```python
from build123d import *

# Parameters (mm, degrees)
MODEL_R         = 1
MODEL_R_2       = 1.05
MODEL_W         = 13.99947
MODEL_H         = 13.99944
MODEL_W_2       = 2.54
MODEL_H_2       = 5.78308735
MODEL_W_3       = 13.9994
MODEL_W_4       = 13.9993
MODEL_H_3       = 13.9993
MODEL_R_3       = 2.032
MODEL_R_4       = 3.048
EXTRUDE_1_DEPTH = 1.5


with BuildPart() as part:
    # Model → 凸台-拉伸1 (new body)
    with BuildSketch(Plane.XY):
        with BuildLine():
            Line((57.046434605, 41.37894176), (0.354810268, 41.37894176))
            ThreePointArc((0.354810268, 41.37894176), (-0.846923686, 40.881370762), (-1.345189448, 39.679924707))
            Line((-1.345189448, 39.679924707), (-1.353515518, 25.280051374))
            Line((-1.353515518, 25.280051374), (-1.356811329, 19.579970423))
            Line((-1.356811329, 19.579970423), (-4.853485523, 18.100805857))
            Line((-4.853485523, 18.100805857), (-4.853710523, 15.920120221))
            Line((-4.853710523, 15.920120221), (-4.853736766, 15.66577888))
            Line((-4.853736766, 15.66577888), (-1.359820188, 14.394107598))
            Line((-1.359820188, 14.394107598), (-1.362991715, 8.917997305))
            Line((-1.362991715, 8.917997305), (-4.9049154, 4.538497879))
            Line((-4.9049154, 4.538497879), (-4.9049154, 3.15597541))
            Line((-4.9049154, 3.15597541), (-4.883883595, 2.639206616))
            Line((-4.883883595, 2.639206616), (-4.813264805, 2.011073476))
            Line((-4.813264805, 2.011073476), (-4.687062167, 1.387481119))
            Line((-4.687062167, 1.387481119), (-4.516803943, 0.776764684))
            Line((-4.516803943, 0.776764684), (-4.295659415, 0.187060206))
            Line((-4.295659415, 0.187060206), (-4.03681533, -0.378036856))
            Line((-4.03681533, -0.378036856), (-3.730362364, -0.921623746))
            Line((-3.730362364, -0.921623746), (-3.390574278, -1.434889052))
            Line((-3.390574278, -1.434889052), (-2.992281832, -1.942165148))
            Line((-2.992281832, -1.942165148), (-2.558331876, -2.409802006))
            Line((-2.558331876, -2.409802006), (-2.102251702, -2.829663369))
            Line((-2.102251702, -2.829663369), (-1.614610519, -3.215411153))
            Line((-1.614610519, -3.215411153), (-1.088890304, -3.567123565))
            Line((-1.088890304, -3.567123565), (-0.532800957, -3.878547051))
            Line((-0.532800957, -3.878547051), (0.038326794, -4.140153507))
            Line((0.038326794, -4.140153507), (0.615600502, -4.353028424))
            Line((0.615600502, -4.353028424), (1.223529929, -4.526191258))
            Line((1.223529929, -4.526191258), (1.847223482, -4.64943937))
            Line((1.847223482, -4.64943937), (2.464503115, -4.722060038))
            Line((2.464503115, -4.722060038), (2.992774524, -4.743685))
            Line((2.992774524, -4.743685), (54.34686609, -4.743685))
            Line((54.34686609, -4.743685), (54.87843401, -4.722059086))
            Line((54.87843401, -4.722059086), (55.492240411, -4.649391053))
            Line((55.492240411, -4.649391053), (56.11599848, -4.526806688))
            Line((56.11599848, -4.526806688), (56.726168878, -4.352867841))
            Line((56.726168878, -4.352867841), (57.302144081, -4.140491025))
            Line((57.302144081, -4.140491025), (57.880206411, -3.875955859))
            Line((57.880206411, -3.875955859), (58.434482529, -3.563431063))
            Line((58.434482529, -3.563431063), (58.947571314, -3.220379587))
            Line((58.947571314, -3.220379587), (59.445938304, -2.8287768))
            Line((59.445938304, -2.8287768), (59.905767444, -2.401934126))
            Line((59.905767444, -2.401934126), (60.332973054, -1.941418241))
            Line((60.332973054, -1.941418241), (60.721224007, -1.446690794))
            Line((60.721224007, -1.446690794), (61.064717919, -0.934798534))
            Line((61.064717919, -0.934798534), (61.379380282, -0.376374826))
            Line((61.379380282, -0.376374826), (61.644240363, 0.202684675))
            Line((61.644240363, 0.202684675), (61.855333273, 0.776565869))
            Line((61.855333273, 0.776565869), (62.029241049, 1.384922025))
            Line((62.029241049, 1.384922025), (62.152356641, 2.011350393))
            Line((62.152356641, 2.011350393), (62.226202972, 2.636734827))
            Line((62.226202972, 2.636734827), (62.245297192, 3.166071528))
            Line((62.245297192, 3.166071528), (58.745412398, 6.86443549))
            Line((58.745412398, 6.86443549), (58.74568075, 14.685402523))
            Line((58.74568075, 14.685402523), (62.245579127, 15.434705638))
            Line((62.245579127, 15.434705638), (62.245861062, 18.167199282))
            Line((62.245861062, 18.167199282), (58.745799684, 19.296928449))
            Line((58.745799684, 19.296928449), (58.745975132, 24.929084585))
            Line((58.745975132, 24.929084585), (58.746434604, 39.678888803))
            ThreePointArc((58.746434604, 39.678888803), (58.248534856, 40.881004565), (57.046434605, 41.37894176))
        make_face()
        with Locations((8.744501265, -2.189788582)):
            Circle(MODEL_R, mode=Mode.SUBTRACT)
        with Locations((19.14575, 5.311768186)):
            Circle(MODEL_R_2, mode=Mode.SUBTRACT)
        with Locations((9.620765, 9.78198)):
            Rectangle(MODEL_W, MODEL_H, mode=Mode.SUBTRACT)
        with Locations((-2.255498735, 16.910211418)):
            Circle(MODEL_R, mode=Mode.SUBTRACT)
        with Locations((19.167580955, 11.605191102)):
            Rectangle(MODEL_W_2, MODEL_H_2, mode=Mode.SUBTRACT)
        with Locations((38.19575, 5.272237591)):
            Circle(MODEL_R_2, mode=Mode.SUBTRACT)
        with Locations((48.744501265, -2.189788582)):
            Circle(MODEL_R, mode=Mode.SUBTRACT)
        with Locations((28.6707, 9.78198)):
            Rectangle(MODEL_W_3, MODEL_H, mode=Mode.SUBTRACT)
        with Locations((47.72075, 9.78198)):
            Rectangle(MODEL_W_4, MODEL_H, mode=Mode.SUBTRACT)
        with Locations((59.944501265, 16.910211418)):
            Circle(MODEL_R, mode=Mode.SUBTRACT)
        with Locations((9.620765, 28.83195)):
            Rectangle(MODEL_W, MODEL_H_3, mode=Mode.SUBTRACT)
        with Locations((19.1458, 28.832)):
            Circle(MODEL_R_3, mode=Mode.SUBTRACT)
        with Locations((0.354810268, 39.67894176)):
            Circle(MODEL_R, mode=Mode.SUBTRACT)
        with Locations((19.14575, 33.310608186)):
            Circle(MODEL_R_2, mode=Mode.SUBTRACT)
        with Locations((28.6708, 28.832)):
            Circle(MODEL_R_4, mode=Mode.SUBTRACT)
        with Locations((38.1958, 28.832)):
            Circle(MODEL_R_3, mode=Mode.SUBTRACT)
        with Locations((47.72075, 28.83195)):
            Rectangle(MODEL_W_4, MODEL_H_3, mode=Mode.SUBTRACT)
        with Locations((38.194579287, 33.311869349)):
            Circle(MODEL_R_2, mode=Mode.SUBTRACT)
        with Locations((57.046434605, 39.67894176)):
            Circle(MODEL_R, mode=Mode.SUBTRACT)
    extrude(amount=EXTRUDE_1_DEPTH)


solid = part.part
```
Read the model definition and answer for the solid it produces. Units are mm, in the model's axes. A direction names the side the tool comes from. Give positions to 0.01 mm unless a question says otherwise; leave off trailing zeros. Loops run counter-clockwise (first coordinate to the right, second up) from the corner with the lowest first, then second, coordinate; pieces in that order, holes last.
Item 1: For faces 5 (the cylindrical face through (58.26, 40.87, 0.74)), 6 (the flat face through (40.721, 29, 1)), 7 (the flat face through (-3.13, 15.04, 0.74)), determine the directions among +Z, -Z, +X, -X, +Y, -Y from which every point of the face is accessible in a straight line to the end or side of a thin tool.
Item 2: The part is cut by section C-C (y = 23.5). Write down the section's boundary in (x, z).
Item 3: The part is cut by section B-B (x = 13.5). Write down the section's boundary in (y, z).
Item 4: Find the intervals of material crossed by line 1 along Y through (x, z) = (41.5, 0.1); line 2 along X through (y, z) = (22.5, 0.6); line 3 along X through (y, z) = (11, 0.25), in increasing order.
Item 5: The part is cut by section D-D (y = 8). Write down the section's boundary in (x, z), and give its area (3 significant figures).
Item 6: The mould has two halves that part along X. Classify faces 1 (the flat face through (60.471, 15.055, 0.74)), 2 (the cylindrical face through (36.7, 30.21, 0.74)), 3 (the cylindrical face through (-0.834, 40.895, 0.74)), 4 (the flat face through (48, 16.782, 1)): released by +X, released by -X, zero draft, split by the parting line, or undercut.
Item 7: This flat-tipped pin is pushed along its axis until it touches: pin 1 Ø0.8 at (y, z) = (12, 0.5) entering from -X. Where does it stop, or does it pass through?
Item 8: The part is cut by section A-A (x = 23.5). Write down the section's boundary in (y, z).
Taken from the geometry:
1. face 5: +Z, -Z, +X, +Y
1. face 6: +Z, -Z
1. face 7: +Z, -Z, -X
2. outline: (-1.35, 0) - (2.62, 0) - (2.62, 1.5) - (-1.35, 1.5) - close; (16.62, 0) - (40.72, 0) - (40.72, 1.5) - (16.62, 1.5) - close; (54.72, 0) - (58.75, 0) - (58.75, 1.5) - (54.72, 1.5) - close
3. outline: (-4.74, 0) - (2.78, 0) - (2.78, 1.5) - (-4.74, 1.5) - close; (16.78, 0) - (21.83, 0) - (21.83, 1.5) - (16.78, 1.5) - close; (35.83, 0) - (41.38, 0) - (41.38, 1.5) - (35.83, 1.5) - close
4. line 1: y = -4.74 to 2.78, 16.78 to 21.83, 35.83 to 41.38
4. line 2: x = -1.36 to 2.62, 16.62 to 40.72, 54.72 to 58.75
4. line 3: x = -1.36 to 2.62, 16.62 to 17.9, 20.44 to 21.67, 35.67 to 40.72, 54.72 to 58.75
5. outline: (-2.11, 0) - (2.62, 0) - (2.62, 1.5) - (-2.11, 1.5) - close; (16.62, 0) - (21.67, 0) - (21.67, 1.5) - (16.62, 1.5) - close; (35.67, 0) - (40.72, 0) - (40.72, 1.5) - (35.67, 1.5) - close; (54.72, 0) - (58.75, 0) - (58.75, 1.5) - (54.72, 1.5) - close
5. area: 28.3 mm2
6. face 1: released by +X
6. face 2: undercut
6. face 3: released by -X
6. face 4: undercut
7. pin 1: stops at x = -1.36
8. outline: (-4.74, 0) - (2.78, 0) - (2.78, 1.5) - (-4.74, 1.5) - close; (16.78, 0) - (41.38, 0) - (41.38, 1.5) - (16.78, 1.5) - close
